Autodesk Inventor part; units mm, degrees
ref_plane "YZ Plane" through (0, 0, 0) normal (1, 0, 0) x (0, 1, 0)
ref_plane "XZ Plane" through (0, 0, 0) normal (0, 1, 0) x (-1, 0, 0)
ref_plane "XY Plane" through (0, 0, 0) normal (0, 0, 1) x (1, 0, 0)
sketch "Sketch1" plane through (0, 0, 0) normal (0, 0, 1) x (1, 0, 0)
  line L0 (-82, -50) -> (82, -50)
  line L1 (82, -50) -> (82, 50)
  line L2 (82, 50) -> (-82, 50)
  line L3 (-82, 50) -> (-82, -50)
  line L4 (-82, -50) -> (82, 50) construction
  line L5 (82, -50) -> (-82, 50) construction
  point P0 (0, 0)
  dimension "d0" = 164
  dimension "d1" = 100
extrude "Extrusion1" add sketch "Sketch1" along normal mid plane 12
sketch "Sketch2" plane through (0, 0, 6) normal (0, 0, 1) x (1, 0, 0)
  line L0 (-82, 50) -> (-82, -50)
  line L1 (-82, -30) -> (-70, -30)
  line L2 (-70, -30) -> (-70, -10)
  line L3 (-70, -10) -> (-82, -10)
  line L4 (-82, -10) -> (-82, -30)
  line L5 (-82, -50) -> (82, -50)
  line L6 (-82, 10) -> (-70, 10)
  line L7 (-70, 10) -> (-70, 30)
  line L8 (-70, 30) -> (-82, 30)
  line L9 (-82, 30) -> (-82, 10)
  point P0 (0, 0)
  dimension "d4" = 12
  dimension "d5" = 20
  dimension "d6" = 20
  dimension "d7" = 20
  dimension "d8" = 20
extrude "Extrusion2" cut sketch "Sketch2" against normal through all
mirror "Mirror1" about plane through (0, 0, 0) normal (1, 0, 0) of "Extrusion2"
sketch "Sketch5" plane through (0, 0, 6) normal (0, 0, 1) x (1, 0, 0)
  circle A0 centre (0, 0) radius 5
  dimension "d17" = 10
extrude "Extrusion4" cut sketch "Sketch5" against normal through all
properties part number "FRONT V2" material "Wood (Cherry)"
Here's how the part is built. I have some questions about the finished solid (model axes, mm). A direction names the side the tool comes from. Coordinates: 2 decimals unless noted, no trailing zeros. Order: outer loops, then holes, each group sorted by start corner. A loop starts at its lowest first (then second) coordinate and runs counter-clockwise, first axis right, second up.
1) Imagine slicing it at D-D on y = -27.5. List the corners of the cut face in (x, z) for me, and give its area (3 significant figures).
2) Which directions (+Z, -Z, +X, -X, +Y, -Y) give clear straight access to the entire face, cutting with the end or side of a thin tool? Please do faces 1 (the face through (76, 30, 0)), 2 (the face through (-1.08, -4.88, 0.08)), 3 (the face through (-70, 20, 0)).
3) I need wall thicknesses on line 1 (Y direction, x = 74, z = 5.25); line 2 (Y direction, x = 0, z = 0.75); line 3 (X direction, y = 15.5, z = -3). Which ranges of each line are inside material? Lowest first, please.
4) Imagine slicing it at B-B on z = -1.25. List the corners of the cut face in (x, y) for me.
5) We'd pull the mould along Y, two halves only. Please class faces 4 (the face through (76, -10, 0)), 5 (the face through (-1, 12, -6)), 6 (the face through (1, 50, 0)), 7 (the face through (70, 20, 0)): +Y half, -Y half, draft (parallel to the pull), parting line (faces both ways), or undercut.
6) Imagine slicing it at C-C on y = 0. List the corners of the cut face in (x, z) for me.
7) Will these pins go through, and if not, where does the flat tip stop? pin 1 (3.5 mm diameter, centred on y = 22.5, z = -2, fed in from -X); pin 2 (9 mm diameter, centred on x = 0, y = 0, fed in from +Z).
8) Imagine slicing it at A-A on x = 0. List the corners of the cut face in (y, z) for me.
Response values:
1. outline: (-70, -6) - (70, -6) - (70, 6) - (-70, 6) - close
1. area: 1,680 mm2
2. face 1: +Z, -Z, +X
2. face 2: +Z, -Z
2. face 3: +Z, -Z, -X
3. line 1: y = -50 to -30, -10 to 10, 30 to 50
3. line 2: y = -50 to -5, 5 to 50
3. line 3: x = -70 to 70
4. outline: (-82, -50) - (82, -50) - (82, -30) - (70, -30) - (70, -10) - (82, -10) - (82, 10) - (70, 10) - (70, 30) - (82, 30) - (82, 50) - (-82, 50) - (-82, 30) - (-70, 30) - (-70, 10) - (-82, 10) - (-82, -10) - (-70, -10) - (-70, -30) - (-82, -30) - close; hole circle Ø10 at (0, 0)
5. face 4: undercut
5. face 5: draft
5. face 6: +Y half
5. face 7: undercut
6. outline: (-82, -6) - (-5, -6) - (-5, 6) - (-82, 6) - close; (5, -6) - (82, -6) - (82, 6) - (5, 6) - close
7. pin 1: stops at x = -70
7. pin 2: passes through
8. outline: (-50, -6) - (-5, -6) - (-5, 6) - (-50, 6) - close; (5, -6) - (50, -6) - (50, 6) - (5, 6) - close
